Check sheet for the modelled part. Datum: model origin and axes. Units: mm. Round coordinates to 2 decimals unless told otherwise and drop trailing zeros. Write each loop counter-clockwise with the first axis right and the second up, starting at its lowest first coordinate (ties: lowest second). Pieces come first, ordered by that corner, then holes. Notation, with made-up numbers: (25.25, 44) - (55.25, 44) arc R18 cw to (55.25, 60) - close; hole circle Ø10 at (69, 64.25). An arc over 180 degrees is marked (long way). Answer as a JSON object with one key per item and string values. Group by question number.
Item 1: Sectioned sample at C-C on z = 87. Record the boundary of the cut face in (x, y).
Item 2: Sectioned sample at B-B on z = 36.5. Record the boundary of the cut face in (x, y).
Item 3: Thickness scan on line 1 (X direction, y = 4.75, z = 79.5); line 2 (X direction, y = 8.5, z = 82); line 3 (X direction, y = 2.45, z = 5.7). Record the ranges inside material, lowest first.
Item 4: Sectioned sample at D-D on x = 61. Record the boundary of the cut face in (y, z), plus the area to 3 significant figures.
Item 5: Sectioned sample at A-A on x = 50. Record the boundary of the cut face in (y, z).
Item 6: Gauge pin test, flat ends, axial feed: P1, Ø1.4, axis at x = 41.5, y = 8, coming from the +Z side; P2, Ø0.7, axis at y = 8, z = 18.5, coming from the -X side; P3, Ø5, axis at x = 44, y = 3, coming from the -Z side; P4, Ø0.5, axis at y = 9, z = 89, coming from the -X side. Record the tip position at first contact, or that the pin passes through.
Autodesk Fusion 360 part; units mm, degrees
sketch "Esboço1" plane through (0, 0, 0) normal (0, 1, 0) x (1, 0, 0)
  line L0 (0, -5) -> (0, -164)
  arc A0 (71, -169) -> (76, -164) centre (71, -164) ccw
  circle A1 centre (67.1121, -163.3) radius 2
  arc A2 (76, -5) -> (71, 0) centre (71, -5) ccw
  line L1 (4, -9.5) -> (72, -9.5)
  circle A3 centre (67.1121, -5.7) radius 2
  arc A4 (5, 0) -> (0, -5) centre (5, -5) ccw
  line L2 (72, -9.5) -> (72, -159.5)
  circle A5 centre (8.8879, -163.3) radius 2
  line L3 (72, -159.5) -> (4, -159.5)
  arc A6 (0, -164) -> (5, -169) centre (5, -164) ccw
  line L4 (76, -164) -> (76, -5)
  circle A7 centre (8.8879, -5.7) radius 2
  line L5 (71, 0) -> (5, 0)
  line L6 (4, -159.5) -> (4, -9.5)
  line L7 (5, -169) -> (71, -169)
extrude "Extrusão1" add sketch "Esboço1" along normal blind 5 contours L0 A0 A2 A4 A6 L4 L5 L7 | L1 L2 L3 L6
sketch "Esboço3" plane through (0, 5, 0) normal (0, 1, 0) x (-1, 0, 0)
  circle A0 centre (-8.8879, 163.3) radius 2
  circle A1 centre (-67.1121, 5.7) radius 2
  circle A2 centre (-67.1121, 163.3) radius 2
  circle A3 centre (-8.8879, 5.7) radius 2
  line L0 (-5, 169) -> (-71, 169)
  arc A4 (-71, 169) -> (-76, 164) centre (-71, 164) ccw
  line L1 (-76, 164) -> (-76, 5)
  arc A5 (-76, 5) -> (-71, 0) centre (-71, 5) ccw
  line L2 (-71, 0) -> (-5, 0)
  arc A6 (-5, 0) -> (0, 5) centre (-5, 5) ccw
  line L3 (0, 5) -> (0, 164)
  arc A7 (0, 164) -> (-5, 169) centre (-5, 164) ccw
  line L4 (-76, 164) -> (-76, 5)
  arc A8 (-5, 0) -> (0, 5) centre (-5, 5) ccw
  circle A9 centre (-8.8879, 5.7) radius 2
  arc A10 (0, 164) -> (-5, 169) centre (-5, 164) ccw
  line L5 (-72, 159.5) -> (-4, 159.5)
  circle A11 centre (-8.8879, 163.3) radius 2
  arc A12 (-71, 169) -> (-76, 164) centre (-71, 164) ccw
  line L6 (-4, 159.5) -> (-4, 9.5)
  circle A13 centre (-67.1121, 5.7) radius 2
  line L7 (-4, 9.5) -> (-72, 9.5)
  arc A14 (-76, 5) -> (-71, 0) centre (-71, 5) ccw
  line L8 (0, 5) -> (0, 164)
  circle A15 centre (-67.1121, 163.3) radius 2
  line L9 (-5, 169) -> (-71, 169)
  line L10 (-72, 9.5) -> (-72, 159.5)
  line L11 (-71, 0) -> (-5, 0)
  line L12 (-71.6, 159.1) -> (-4.4, 159.1)
  line L13 (-4.4, 159.1) -> (-4.4, 9.9)
  line L14 (-4.4, 9.9) -> (-71.6, 9.9)
  line L15 (-71.6, 9.9) -> (-71.6, 159.1)
  point P0 (-76, 169)
  dimension "d3" = 0.4
extrude "Extrusão2" add sketch "Esboço3" along normal blind 2 contours L12 L13 L14 L15
sketch "Esboço4" plane through (0, 7, 0) normal (0, 1, 0) x (-1, 0, 0)
  line L0 (-71.6, 9.9) -> (-4.4, 9.9)
  line L1 (-4.4, 9.9) -> (-4.4, 159.1)
  line L2 (-4.4, 159.1) -> (-71.6, 159.1)
  line L3 (-71.6, 159.1) -> (-71.6, 9.9)
  line L4 (-52.7, 24.8) -> (-52.7, 83)
  line L5 (-35.5, 24.2) -> (-41.5, 24.2)
  line L6 (-24.3, 24.8) -> (-35.5, 24.8)
  line L7 (-41.5, 24.2) -> (-41.5, 24.8)
  line L8 (-24.3, 83) -> (-24.3, 24.8)
  line L9 (-52.7, 83) -> (-41.5, 83)
  line L10 (-41.5, 24.8) -> (-52.7, 24.8)
  line L11 (-41.5, 83.6) -> (-35.5, 83.6)
  line L12 (-35.5, 83.6) -> (-35.5, 83)
  line L13 (-35.5, 83) -> (-24.3, 83)
  line L14 (-41.5, 83) -> (-41.5, 83.6)
  line L15 (-35.5, 24.8) -> (-35.5, 24.2)
  line L16 (-29.6883, 89.4117) -> (-29.6883, 88.8117)
  line L17 (-29.6883, 88.8117) -> (-18.4883, 88.8117)
  line L18 (-18.4883, 88.8117) -> (-18.4883, 18.9883)
  line L19 (-18.4883, 18.9883) -> (-29.6883, 18.9883)
  line L20 (-29.6883, 18.9883) -> (-29.6883, 18.3883)
  line L21 (-29.6883, 18.3883) -> (-47.3117, 18.3883)
  line L22 (-47.3117, 18.3883) -> (-47.3117, 18.9883)
  line L23 (-47.3117, 18.9883) -> (-58.5117, 18.9883)
  line L24 (-58.5117, 18.9883) -> (-58.5117, 88.8117)
  line L25 (-58.5117, 88.8117) -> (-47.3117, 88.8117)
  line L26 (-47.3117, 88.8117) -> (-47.3117, 89.4117)
  line L27 (-47.3117, 89.4117) -> (-29.6883, 89.4117)
  dimension "d6" = -5.8117
extrude "Extrusão3" add sketch "Esboço4" along normal blind 2.8 contours L16 L17 L18 L19 L20 L21 L22 L23 L24 L25 L26 L27
extrude "Extrusão4" cut 1 faces at (48.9667, 7, 44.2) along direction (0, -1, 0) blind 14
sketch "Esboço5" plane through (0, 0, 83.6) normal (0, 0, -1) x (-1, 0, 0)
  line L0 (-35.5, 0) -> (-35.5, 9.8)
  line L1 (-35.5, 9.8) -> (-41.5, 9.8)
  line L2 (-41.5, 9.8) -> (-41.5, 0)
  line L3 (-41.5, 0) -> (-35.5, 0)
  line L4 (-35.5, 4.9) -> (-36, 4.9)
  line L5 (-36, 4.9) -> (-41.5, 4.9)
  line L6 (-35.5, 5) -> (-36, 5)
  line L7 (-36, 5) -> (-41.5, 5)
  line L8 (-35.5, 4.8) -> (-36, 4.8)
  line L9 (-36, 4.8) -> (-41.5, 4.8)
  dimension "d11" = 0.1
  dimension "d12" = -0.1
extrude "Extrusão5" cut sketch "Esboço5" against normal blind 0.3 contours L0 L2 L4 L5 L8 L9 | L0 L2 L4 L5 L6 L7
chamfer "Chanfro1" distance 1.2 distance2 0.3 1 edges at (38.5, 5, 83.6) measured on face at (39.5, 8.2, 83.6)
chamfer "Chanfro2" distance 1.2 distance2 0.3 1 edges at (38.5, 4.8, 83.6) measured on face at (39.5, 3.2, 83.6)
sketch "Esboço6" plane through (0, 0, 24.2) normal (0, 0, 1) x (1, 0, 0)
  line L0 (41.5, 0) -> (41.5, 9.8)
  line L1 (41.5, 9.8) -> (35.5, 9.8)
  line L2 (35.5, 9.8) -> (35.5, 0)
  line L3 (35.5, 0) -> (41.5, 0)
  line L4 (35.5, 4.9) -> (41.5, 4.9)
  line L5 (35.5, 4.8) -> (41.5, 4.8)
  line L6 (35.5, 5) -> (41.5, 5)
  dimension "d19" = 0.1
  dimension "d20" = -0.1
extrude "Extrusão6" cut sketch "Esboço6" against normal blind 0.3 contours L0 L2 L4 L5 | L0 L2 L4 L6
chamfer "Chanfro3" distance 1.2 distance2 0.3 1 edges at (38.5, 5, 24.2) measured on face at (37.5, 8.2, 24.2)
chamfer "Chanfro4" distance 1.2 distance2 0.3 1 edges at (38.5, 4.8, 24.2) measured on face at (37.5, 3.2, 24.2)
fillet "Arredondamento1" radius 3 8 edges at (0, 0, 84.5) (1.4645, 0, 167.5355) (38, 0, 169) (74.5355, 0, 167.5355) (76, 0, 84.5) (74.5355, 0, 1.4645) (38, 0, 0) (1.4645, 0, 1.4645)
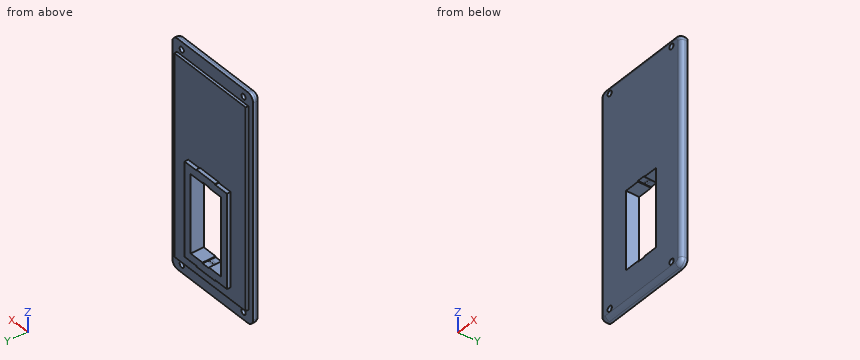
Completed:
{
 "1": {"outline": "(0, 3) arc R3 ccw to (3, 0) - (73, 0) arc R3 ccw to (76, 3) - (76, 5) - (71.6, 5) - (71.6, 7) - (58.51, 7) - (58.51, 9.8) - (18.49, 9.8) - (18.49, 7) - (4.4, 7) - (4.4, 5) - (0, 5) - close"},
 "2": {"outline": "(0, 3) arc R3 ccw to (3, 0) - (24.3, 0) - (24.3, 9.8) - (18.49, 9.8) - (18.49, 7) - (4.4, 7) - (4.4, 5) - (0, 5) - close; (52.7, 0) - (73, 0) arc R3 ccw to (76, 3) - (76, 5) - (71.6, 5) - (71.6, 7) - (58.51, 7) - (58.51, 9.8) - (52.7, 9.8) - close"},
 "3": {"line 1": "0 to 24.3, 52.7 to 76", "line 2": "18.49 to 24.3, 52.7 to 58.51", "line 3": "0.05 to 6.89, 10.89 to 65.11, 69.11 to 75.95"},
 "4": {"outline": "(0, 3) arc R3 ccw to (3, 0) - (5, 0) - (5, 9.9) - (7, 9.9) - (7, 159.1) - (5, 159.1) - (5, 169) - (3, 169) arc R3 ccw to (0, 166) - close", "area": "1,140 mm²"},
 "5": {"outline": "(0, 3) arc R3 ccw to (3, 0) - (5, 0) - (5, 9.9) - (7, 9.9) - (7, 18.99) - (9.8, 18.99) - (9.8, 24.8) - (0, 24.8) - close; (0, 83) - (9.8, 83) - (9.8, 88.81) - (7, 88.81) - (7, 159.1) - (5, 159.1) - (5, 169) - (3, 169) arc R3 ccw to (0, 166) - close"},
 "6": {"P1": "z = 89.41", "P2": "x = 29.69", "P3": "z = 0", "P4": "x = 18.49"}
}
